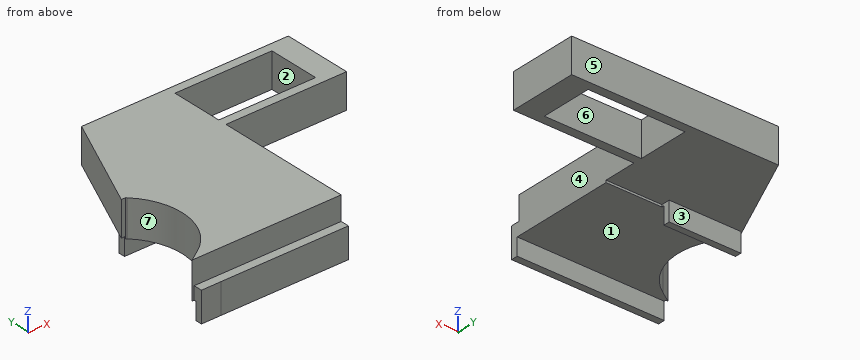
from build123d import *

# Parameters (mm, degrees)
F0_W     = 22.5
F0_H     = 12
F0_W_2   = 16.6362704164
F0_H_2   = 1.4672726393
F1_DEPTH = 8.5
F0_W_3   = 12.9140389063
F0_H_3   = 0.4558046321
F0_H_4   = 1.5437308085
F2_DEPTH = 3
F3_DEPTH = 4
F4_DEPTH = 0.5
F5_DEPTH = 0.5
F6_DEPTH = 4


# Not quite as in the source:
# - a feature names something its author has since deleted; it is built from what else it names


with BuildPart() as f1:
    # F0 (on Top) → F1 (new body)
    with BuildSketch(Plane.XY):
        Polygon((-28.1854607165, -113.3383650622), (-15.2103829287, -113.3383650622), (-15.2103829287, -112.8061022609), (-15.2103829287, -111.3388296217), (-15.2103829287, -105.6495462671), (-21.261529997, -105.6495462671), (-21.261529997, -89.6495462671), (-35.2103829287, -89.6495462671), (-46.0062867338, -113.3383650622), (-45.0214308559, -113.3383650622), (-44.8217311329, -113.3383650622), (-44.8217311329, -112.8061022609), (-44.8217311329, -111.3388296217), (-28.1854607165, -111.3388296217), (-28.1854607165, -112.8061022609), align=None)
        Polygon((-28.1244218349, -137.2695039054), (-15.2103829287, -137.2695039054), (-15.2103829287, -136.6045172354), (-15.2103829287, -114.0332519535), (-15.2103829287, -113.3383650622), (-28.1854607165, -113.3383650622), (-35.2103829287, -113.3383650622), (-35.2103829287, -125.3039344838), (-35.2103829287, -137.2695039054), align=None)
        with BuildLine():
            Line((-49.3365414441, -137.2695039054), (-35.2103829287, -137.2695039054))
            Line((-35.2103829287, -137.2695039054), (-35.2103829287, -125.3039344838))
            Line((-35.2103829287, -125.3039344838), (-35.2103829287, -113.3383650622))
            Line((-35.2103829287, -113.3383650622), (-44.8217311329, -113.3383650622))
            Line((-44.8217311329, -113.3383650622), (-44.8217311329, -113.5371806076))
            ThreePointArc((-44.8217311329, -113.5371806076), (-40.72117222, -125.1132769851), (-47.1813260123, -135.5577493852))
            Line((-47.1813260123, -135.5577493852), (-49.8537484313, -137.2695039054))
            Line((-49.8537484313, -137.2695039054), (-49.3365414441, -137.2695039054))
        make_face()
        Polygon((-21.261529997, -105.6495462671), (-15.2103829287, -105.6495462671), (7.2896170713, -105.6495462671), (12.7896170713, -105.6495462671), (12.7896170713, -91.6495462671), (12.7896170713, -89.6495462671), (-15.2103829287, -89.6495462671), (-21.261529997, -89.6495462671), align=None)
        with Locations((-3.9603829287, -97.6495462671)):
            Rectangle(F0_W, F0_H, mode=Mode.SUBTRACT)
        Polygon((-35.2103829287, -113.3383650622), (-28.1854607165, -113.3383650622), (-28.1854607165, -112.8061022609), (-44.8217311329, -112.8061022609), (-44.8217311329, -113.3383650622), align=None)
        with Locations((-36.5035959247, -112.0724659413)):
            Rectangle(F0_W_2, F0_H_2)
        Polygon((-44.8217311329, -113.5371806076), (-44.8217311329, -113.3383650622), (-45.0214308559, -113.3383650622), align=None)
    extrude(amount=F1_DEPTH)

    # F0 (on Top) → F2 (join)
    with BuildSketch(Plane.XY):
        Polygon((-28.1244218349, -137.7253085375), (-28.1244218349, -137.2695039054), (-35.2103829287, -137.2695039054), (-49.3365414441, -137.2695039054), (-49.3365414441, -137.7253085375), align=None)
        Polygon((-28.1244218349, -139.269039346), (-28.1244218349, -137.7253085375), (-49.3365414441, -137.7253085375), (-49.3365414441, -139.2803862691), (-44.8217311329, -139.269039346), align=None)
        with Locations((-21.6674023818, -137.4974062214)):
            Rectangle(F0_W_3, F0_H_3)
        with Locations((-21.6674023818, -138.4971739417)):
            Rectangle(F0_W_3, F0_H_4)
    extrude(amount=F2_DEPTH)

    # F0 (on Top) → F3 (join)
    with BuildSketch(Plane.XY):
        Polygon((-28.1244218349, -139.269039346), (-28.1244218349, -137.7253085375), (-49.3365414441, -137.7253085375), (-49.3365414441, -139.2803862691), (-44.8217311329, -139.269039346), align=None)
        with Locations((-21.6674023818, -138.4971739417)):
            Rectangle(F0_W_3, F0_H_4)
    extrude(amount=-F3_DEPTH)

    # F0 (on Top) → F4 (cut)
    with BuildSketch(Plane.XY):
        Polygon((-28.1854607165, -113.3383650622), (-15.2103829287, -113.3383650622), (-15.2103829287, -112.8061022609), (-15.2103829287, -111.3388296217), (-15.2103829287, -105.6495462671), (-21.261529997, -105.6495462671), (-21.261529997, -89.6495462671), (-35.2103829287, -89.6495462671), (-46.0062867338, -113.3383650622), (-45.0214308559, -113.3383650622), (-44.8217311329, -113.3383650622), (-44.8217311329, -112.8061022609), (-44.8217311329, -111.3388296217), (-28.1854607165, -111.3388296217), (-28.1854607165, -112.8061022609), align=None)
        Polygon((-21.261529997, -105.6495462671), (-15.2103829287, -105.6495462671), (7.2896170713, -105.6495462671), (12.7896170713, -105.6495462671), (12.7896170713, -91.6495462671), (12.7896170713, -89.6495462671), (-15.2103829287, -89.6495462671), (-21.261529997, -89.6495462671), align=None)
        with Locations((-3.9603829287, -97.6495462671)):
            Rectangle(F0_W, F0_H, mode=Mode.SUBTRACT)
    extrude(amount=F4_DEPTH, mode=Mode.SUBTRACT)

    # F0 (on Top) → F5 (join)
    with BuildSketch(Plane.XY):
        with Locations((-36.5035959247, -112.0724659413)):
            Rectangle(F0_W_2, F0_H_2)
        Polygon((-35.2103829287, -113.3383650622), (-28.1854607165, -113.3383650622), (-28.1854607165, -112.8061022609), (-44.8217311329, -112.8061022609), (-44.8217311329, -113.3383650622), align=None)
    extrude(amount=F5_DEPTH)

    # F0 (on Top) → F6 (join)
    with BuildSketch(Plane.XY):
        with Locations((-36.5035959247, -112.0724659413)):
            Rectangle(F0_W_2, F0_H_2)
    extrude(amount=-F6_DEPTH)


solid = f1.part
Part model, mm, in its own coordinate system. Face numbers are marked on the shaded views. A direction names the side the tool comes from. Round coordinates to 2 decimals unless told otherwise and drop trailing zeros. Order: outer loops, then holes, each group sorted by start corner. A loop starts at its lowest first (then second) coordinate and runs counter-clockwise, first axis right, second up. Notation, with made-up numbers: (12.25, 18) -> (44.25, 18) arc R21 ccw to (44.25, 54) -> close; hole circle Ø8 at (53.5, 58). An arc over 180 degrees is marked (long way). Put each result on its own line as item: value.
Q1. Pin check, flat tips, straight feed: pin 1 Ø7.5 at (x, z) = (-34, -1.5) entering from -Y; pin 2 Ø8 at (x, y) = (-41.5, -125) entering from -Z; pin 3 Ø4 at (y, z) = (-126.5, -0.5) entering from +X. Stop position of each tip, or through.
From the geometry:
pin 1: stops at y = -139.27
pin 2: stops at z = 0
pin 3: stops at x = -15.21
Q2. Band-saw the part on B-B (x = -1). Give the cut face in (y, z).
From the geometry:
outline: (-105.65, 0.5) -> (-103.65, 0.5) -> (-103.65, 8.5) -> (-105.65, 8.5) -> close; (-91.65, 0.5) -> (-89.65, 0.5) -> (-89.65, 8.5) -> (-91.65, 8.5) -> close
Q3. Band-saw the part on C-C (z = -2.25). Give the cut face in (x, y).
From the geometry:
outline: (-49.34, -139.28) -> (-44.82, -139.27) -> (-15.21, -139.27) -> (-15.21, -137.73) -> (-49.34, -137.73) -> close; (-44.82, -112.81) -> (-28.19, -112.81) -> (-28.19, -111.34) -> (-44.82, -111.34) -> close
Q4. Wall check: line 1 (Y direction, x = 6.5, z = 8); line 2 (Y direction, x = -34, z = -2.25); line 3 (Y direction, x = -22, z = 7). Give the ranges that are in metal, low to high. Write a range as [from, to].
From the geometry:
line 1: y = [-105.65, -103.65], [-91.65, -89.65]
line 2: y = [-139.27, -137.73], [-112.81, -111.34]
line 3: y = [-137.27, -89.65]
Q5. Pull direction X, two halves, no side cores. Call the marked faces 5, 6 and 7: pulls with the +X half, pulls with the -X half, needs draft (parallel to the pull), parting line crosses it, or undercut.
From the geometry:
face 5: needs draft
face 6: undercut
face 7: pulls with the -X half
Q6. Band-saw the part on D-D (x = -21). Give the cut face in (y, z).
From the geometry:
outline: (-139.27, -4) -> (-137.73, -4) -> (-137.73, 0) -> (-113.34, 0) -> (-113.34, 0.5) -> (-89.65, 0.5) -> (-89.65, 8.5) -> (-137.27, 8.5) -> (-137.27, 3) -> (-139.27, 3) -> close
Q7. Band-saw the part on A-A (z = 7.25). Give the cut face in (x, y).
From the geometry:
outline: (-49.85, -137.27) -> (-15.21, -137.27) -> (-15.21, -105.65) -> (12.79, -105.65) -> (12.79, -89.65) -> (-35.21, -89.65) -> (-46.01, -113.34) -> (-45.02, -113.34) -> (-44.82, -113.54) arc R14.2 cw to (-47.18, -135.56) -> close; hole (-15.21, -103.65) -> (7.29, -103.65) -> (7.29, -91.65) -> (-15.21, -91.65) -> close
Q8. Tool access for the marked faces 1, 2, 3 and 4: list every direction of +Z, -Z, +X, -X, +Y, -Y with a clear straight run to the whole face (end or side of a thin tool).
From the geometry:
face 1: -Z, +X, -X
face 2: +Z, -Z
face 3: -Z, +X, -X, +Y
face 4: +Z, -Z, +X, -Y
